from build123d import *

# Parameters (mm, degrees)
F0_R     = 2.032
F1_DEPTH = 12.7
F3_D     = 1.778
F3_DEPTH = 5.1707142857
F3_TIP   = 0.5341650903
F5_D     = 1.778
F5_DEPTH = 5.1816
F5_TIP   = 0.5341650903


with BuildPart() as f1:
    # F0 (on Right) → F1 (new body, symmetric)
    with BuildSketch(Plane.YZ):
        Circle(F0_R)
    extrude(amount=F1_DEPTH, both=True)

    # F3
    with Locations(Plane.YZ.offset(12.7)):
        with Locations((0, 0)):
            Hole(F3_D / 2, depth=F3_DEPTH)
            with Locations((0, 0, -(F3_DEPTH + F3_TIP / 2))):  # 118° drill point
                Cone(0, F3_D / 2, F3_TIP, mode=Mode.SUBTRACT)

    # F5
    with Locations(Plane(origin=(-12.7, 0, 0), x_dir=(0, -1, 0), z_dir=(-1, 0, 0))):
        with Locations((0, 0)):
            Hole(F5_D / 2, depth=F5_DEPTH)
            with Locations((0, 0, -(F5_DEPTH + F5_TIP / 2))):  # 118° drill point
                Cone(0, F5_D / 2, F5_TIP, mode=Mode.SUBTRACT)


solid = f1.part
The listing builds one solid part. Answer for the finished solid, in the listing's coordinates (mm). A direction names the side the tool comes from. Round coordinates to 2 decimals unless told otherwise and drop trailing zeros. Loops run counter-clockwise (first coordinate to the right, second up) from the corner with the lowest first, then second, coordinate; pieces in that order, holes last. Notation, with made-up numbers: M -7.75,40 L 9.25,40 A28 cw 9.25,69 Z; hole C -20.5,-14 d8. An arc over 180 degrees is marked long. Write each question's results on one line, items separated by ' | '. Start each with the question number.
1) Straight lines are drawn through the part: probe 1 along Z at (x, y) = (-10.75, 0); probe 2 along Z at (x, y) = (-8.25, -0.5); probe 3 along Y at (x, z) = (-10.5, 0.15). For each, find the intervals that lie inside material, in ascending order.
2) Find section B-B on x = 4.75. Write down the section's boundary in (y, z), plus the area to 3 significant figures.
3) Find section A-A on x = 10.5. Write down the section's boundary in (y, z), plus the area to 3 significant figures.
4) Which of the six approach directions +Z, -Z, +X, -X, +Y, -Y give full straight-line access (tool end or side, diameter ignored) to faces 1 (the cylindrical face through (10.08, 0.19, -0.87)), 2 (the cylindrical face through (-10.07, -0.19, -0.87))?
5) Determine the mould class of faces 3 (the conical face through (7.09, 0.07, -0.14)), 4 (the cylindrical face through (0.178, -0.44, -1.984)) for opening direction Y: pulls with the +Y half, pulls with the -Y half, needs draft (parallel to the pull), parting line crosses it, or undercut.
Final values:
1) probe 1: -2.03 to -0.89, 0.89 to 2.03 | probe 2: -1.97 to -0.74, 0.74 to 1.97 | probe 3: -2.03 to -0.88, 0.88 to 2.03
2) outline: C 0,0 d4.06 | area: 13.0 mm²
3) outline: C 0,0 d4.06; hole C 0,0 d1.78 | area: 10.5 mm²
4) face 1: +X | face 2: -X
5) face 3: undercut | face 4: parting line crosses it
